```python
from build123d import *

# Parameters (mm, degrees)
F1_DEPTH = 63.5
F0_W     = 25.4964783202
F0_H     = 19.05
F2_DEPTH = 25.4
F3_DEPTH = 7.9375
F4_DEPTH = 25.4
F6_R     = 6.35


with BuildPart() as f1:
    # F0 (on Front) → F1 (new body, symmetric)
    with BuildSketch(Plane.XZ):
        Polygon((-41.275, -9.525), (41.275, -9.525), (41.275, 9.525), (22.225, 9.525), (-41.275, 9.525), align=None)
    extrude(amount=F1_DEPTH, both=True)

    # F0 (on Front) → F2 (join, symmetric)
    with BuildSketch(Plane.XZ):
        with BuildLine():
            Line((22.225, 9.525), (41.275, 9.525))
            Line((41.275, 9.525), (41.275, 27.0002))
            ThreePointArc((41.275, 27.0002), (45.9246798487, 38.2255201513), (57.15, 42.8752))
            Line((57.15, 42.8752), (60.325, 42.8752))
            Line((60.325, 42.8752), (60.325, 61.9252))
            Line((60.325, 61.9252), (57.15, 61.9252))
            ThreePointArc((57.15, 61.9252), (32.4542956671, 51.6959043329), (22.225, 27.0002))
            Line((22.225, 27.0002), (22.225, 9.525))
        make_face()
        with Locations((73.0732391601, 52.4002)):
            Rectangle(F0_W, F0_H)
    extrude(amount=F2_DEPTH, both=True)

    # F0 (on Front) → F3 (join, symmetric)
    with BuildSketch(Plane.XZ):
        with BuildLine():
            add(Edge.make_bspline(
                [(-41.275, 9.525), (-41.1518029869, 33.0162532628), (17.5662990659, 62.1782578528), (57.15, 61.9252)],
                knots=[0, 0, 0, 0, 111.5045361635, 111.5045361635, 111.5045361635, 111.5045361635], degree=3))
            Line((-41.275, 9.525), (22.225, 9.525))
            Line((22.225, 9.525), (22.225, 27.0002))
            ThreePointArc((22.225, 27.0002), (32.4542956671, 51.6959043329), (57.15, 61.9252))
        make_face()
    extrude(amount=F3_DEPTH, both=True)

    # F0 (on Front) → F4 (join)
    with BuildSketch(Plane.XZ):
        Polygon((-41.275, -9.525), (41.275, -9.525), (41.275, 9.525), (22.225, 9.525), (-41.275, 9.525), align=None)
    extrude(amount=F4_DEPTH)

    # F0 (on Front) → F5 (revolve)
    with BuildSketch(Plane.XZ):
        Polygon((85.8214783202, 66.675), (85.8214783202, 61.9252), (85.8214783202, 42.8752), (85.8214783202, 38.1), (111.125, 38.1), (111.125, 66.675), align=None)
    revolve(axis=Axis((85.8214783202, 0, 52.3875), (0, 0, 1)))

    # F6
    f6_edges = [f1.edges().sort_by_distance(p)[0] for p in [
        (-41.275, -63.5, 0),
        (41.275, -63.5, 0),
        (-41.275, 63.5, 0),
        (41.275, 63.5, 0),
    ]]
    fillet(f6_edges, radius=F6_R)


solid = f1.part
```
The model under review builds one solid part; all positions refer to its coordinate system, in mm. A direction names the side the tool comes from. Round coordinates to 2 decimals unless told otherwise and drop trailing zeros. Loops run counter-clockwise (first coordinate to the right, second up) from the corner with the lowest first, then second, coordinate; pieces in that order, holes last.
1) Consider section B-B on y = 18.5. State the section outline as (x, z) points (3 decimals).
Values follow:
outline: (-41.275, -9.525) - (41.275, -9.525) - (41.275, 27) arc R15.875 cw to (57.15, 42.875) - (68.558, 42.875) - (68.558, 38.1) - (103.085, 38.1) - (103.085, 66.675) - (68.558, 66.675) - (68.558, 61.925) - (57.15, 61.925) arc R34.925 ccw to (22.225, 27) - (22.225, 9.525) - (-41.275, 9.525) - close
2) Consider section C-C on x = 71. State the section outline as (y, z) points (3 decimals), then the cut area to 3 significant figures.
Values follow:
outline: (-25.4, 42.875) - (-20.508, 42.875) - (-20.508, 38.1) - (20.508, 38.1) - (20.508, 42.875) - (25.4, 42.875) - (25.4, 61.925) - (20.508, 61.925) - (20.508, 66.675) - (-20.508, 66.675) - (-20.508, 61.925) - (-25.4, 61.925) - close
area: 1,360 mm2
3) Clearance check with flat-ended pins moving along their axes: P1, Ø10, axis at x = -20.5, z = 19, coming from the +Y side; P2, Ø15.5, axis at x = 28.5, z = 29.5, coming from the +Y side; P3, Ø5, axis at y = -12.5, z = 15, coming from the -X side (3 decimals); P4, Ø8, axis at x = 92, z = 34, coming from the -Y side. State where each tip first meets the part, or that it passes through.
Values follow:
P1: stops at y = 7.94
P2: stops at y = 25.4
P3: stops at x = 22.225
P4: passes through
4) Wall thickness on line 1 along Y through (x, z) = (-15, 14); line 2 along Y through (x, z) = (40, 46); line 3 along Z through (x, y) = (18.5, 21) (3 decimals): over which ranges is each line inside the solid? List them lowest first.
Values follow:
line 1: y = -7.94 to 7.94
line 2: y = -25.4 to 25.4
line 3: z = -9.525 to 9.525
5) Tool access review of faces 4 (the face through (60, -2, 42.875)), 5 (the face through (-2, -7.938, 30)), 6 (the face through (47, 25.4, 42)), 7 (the face through (47, -25.4, 42)): name each direction out of +Z, -Z, +X, -X, +Y, -Y from which nothing blocks a thin tool from reaching the whole face with its end or side.
Values follow:
face 4: -Z
face 5: +Z, -X, -Y
face 6: +Z, +X, -X, +Y
face 7: +Z, +X, -X, -Y
6) The part is to be moulded in two halves that separate along X. For faces 1 (the face through (45.8, -0.4, 38.1)), 2 (the face through (22.225, 17, 18)), 3 (the face through (85, 0, 66.675)), say which applies: pulls with the +X half, pulls with the -X half, needs draft (parallel to the pull), parting line crosses it, or undercut.
Values follow:
face 1: undercut
face 2: pulls with the -X half
face 3: needs draft
7) Consider section D-D on y = 50.5. State the section outline as (x, z) points (3 decimals).
Values follow:
outline: (-41.275, -9.525) - (41.275, -9.525) - (41.275, 9.525) - (-41.275, 9.525) - close
8) Consider section A-A on z = 1. State the section outline as (x, y) points (3 decimals).
Values follow:
outline: (-41.275, -57.15) arc R6.35 ccw to (-34.925, -63.5) - (34.925, -63.5) arc R6.35 ccw to (41.275, -57.15) - (41.275, 57.15) arc R6.35 ccw to (34.925, 63.5) - (-34.925, 63.5) arc R6.35 ccw to (-41.275, 57.15) - close
